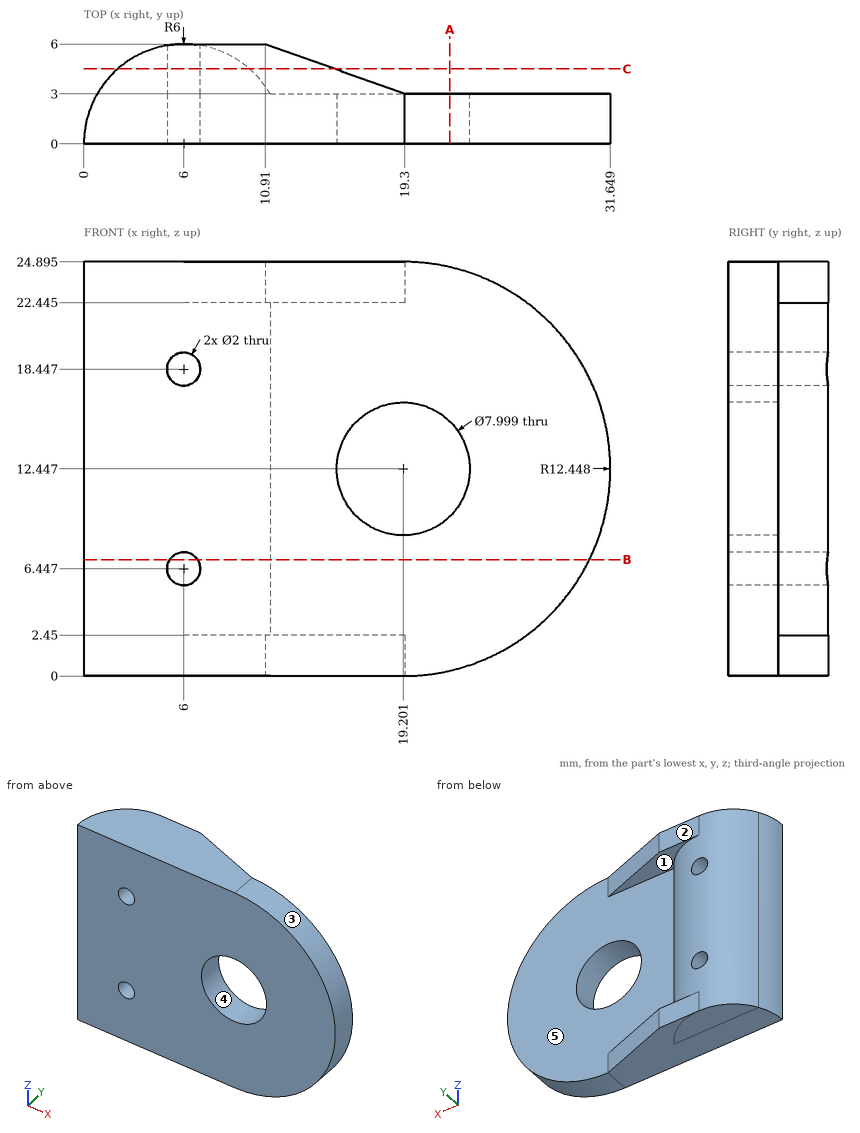
Check sheet for the drawn part. Datum: minimum x, y, z corner. Units: mm. A direction names the side the tool comes from. Coordinates: 2 decimals unless noted, no trailing zeros. Order: outer loops, then holes, each group sorted by start corner. A loop starts at its lowest first (then second) coordinate and runs counter-clockwise, first axis right, second up. Notation, with made-up numbers: M 26,45.25 L 43,45.25 A18 ccw 43,74.25 Z; hole C -31.75,40.5 d4. An arc over 180 degrees is marked long. One line per item, written item: value. Start each with the question number.
Item 1: Access from +Z, -Z, +X, -X, +Y, -Y to the whole of each face (thin tool, end or side, straight path). Record for the marked faces 1 and 2.
Item 2: Gauge pin test, flat ends, axial feed: pin 1 (2 mm diameter, centred on y = 1.5, z = 17, fed in from +X); pin 2 (1.5 mm diameter, centred on y = 4, z = 6.5, fed in from -X) (1 decimal); pin 3 (4 mm diameter, centred on x = 15, z = 3.5, fed in from +Y). Record the tip position at first contact, or that the pin passes through.
Item 3: Scan lines: probe 1 along Z at (x, y) = (6, 2.25) (1 decimal); probe 2 along Y at (x, z) = (24.5, 10.75); probe 3 along X at (y, z) = (1.25, 7) (1 decimal). Record each from-to range of solid material in increasing order.
Item 4: Sectioned sample at C-C (y = 4.5). Count the separate pieces of the cut face and the enclosed holes in it.
Item 5: Sectioned sample at A-A (x = 22). Enter the section's corners in (y, z).
Item 6: Mould release check, pull along X, two halves, no side actions. Record for the marked faces 3, 4 and 5: released by +X, released by -X, zero draft, split by the parting line, or undercut.
Item 7: Sectioned sample at B-B (z = 7). Enter the section's corners in (x, y).
Conclusion:
1. face 1: +X, +Y
1. face 2: +Z, -Z, +X, -X, +Y
2. pin 1: stops at x = 31.13
2. pin 2: stops at x = 1
2. pin 3: stops at y = 5.15
3. probe 1: z = 0 to 5.4, 7.4 to 17.4, 19.4 to 24.9
3. probe 2: y = 0 to 3
3. probe 3: x = 0.1 to 5.2, 6.8 to 30.4
4. separate pieces: 1
4. enclosed holes: 2
5. outline: M 0,0.32 L 3,0.32 L 3,9.59 L 0,9.59 Z; M 0,15.3 L 3,15.3 L 3,24.58 L 0,24.58 Z
6. face 3: released by +X
6. face 4: undercut
6. face 5: zero draft
7. outline: M 0,0 L 5.17,0 L 5.17,5.94 A6 ccw Z; M 6.83,0 L 30.39,0 L 30.39,3 L 11.2,3 A6 ccw 6.83,5.94 Z
